Design review of the part built by this model. Coordinates are the model's own, in mm. A direction names the side the tool comes from. Round coordinates to 2 decimals unless told otherwise and drop trailing zeros. Order: outer loops, then holes, each group sorted by start corner. A loop starts at its lowest first (then second) coordinate and runs counter-clockwise, first axis right, second up.
from build123d import *

# Parameters (mm, degrees)
CROQUIS1_W              = 57
CROQUIS1_H              = 57
SALIENTE_EXTRUIR1_DEPTH = 18
REDONDEO1_R             = 5
CROQUIS2_W              = 14
CROQUIS2_H              = 10
CORTAR_EXTRUIR1_DEPTH   = 5


with BuildPart() as part:
    # Croquis1 → Saliente-Extruir1 (new body)
    with BuildSketch(Plane(origin=(0, 0, 0), x_dir=(1, 0, 0), z_dir=(0, 1, 0))):
        Rectangle(CROQUIS1_W, CROQUIS1_H)
    extrude(amount=SALIENTE_EXTRUIR1_DEPTH)

    # Redondeo1
    redondeo1_edges = [part.edges().sort_by_distance(p)[0] for p in [
        (-28.5, 9, -28.5),
        (28.5, 9, -28.5),
        (28.5, 9, 28.5),
        (-28.5, 9, 28.5),
    ]]
    fillet(redondeo1_edges, radius=REDONDEO1_R)

    # Croquis2 → Cortar-Extruir1 (cut)
    with BuildSketch(Plane(origin=(28.5, 0, 0), x_dir=(0, 0, -1), z_dir=(1, 0, 0))):
        with BuildLine():
            Line((-13, 12.5), (-7, 12.5))
            ThreePointArc((-7, 12.5), (-3.5, 9), (-7, 5.5))
            Line((-7, 5.5), (-13, 5.5))
            ThreePointArc((-13, 5.5), (-16.5, 9), (-13, 12.5))
        make_face()
        with Locations((10.5, 9)):
            Rectangle(CROQUIS2_W, CROQUIS2_H)
    extrude(amount=-CORTAR_EXTRUIR1_DEPTH, mode=Mode.SUBTRACT)


solid = part.part
1) Clearance check with flat-ended pins moving along their axes: P1, Ø1.5, axis at x = 26, y = 11, coming from the +Z side; P2, Ø3.5, axis at y = 10.5, z = 11, coming from the +X side; P3, Ø4, axis at x = 26.5, z = -12.5, coming from the -Y side; P4, Ø2.5, axis at x = 25.5, y = 11, coming from the -Z side. State where each tip first meets the part, or that it passes through.
Results:
P1: stops at z = 28.18
P2: stops at x = 23.5
P3: stops at y = 0
P4: stops at z = -28.44
2) For faces 1 (the face through (26, 8.9, 16.5)), 2 (the face through (0, 9, 28.5)), list the 3-axis set-ups (+Z, -Z, +X, -X, +Y, -Y) from which the entire face can be reached by the end or side of a thin tool; tool diameter is ignored.
Results:
face 1: +X
face 2: +Z, +X, -X, +Y, -Y
3) To check wall thickness, follow line 1 along X through (y, z) = (12, 11.5); line 2 along Z through (x, y) = (-25, 13.75); line 3 along Z through (x, y) = (24, 4.25). State the ranges of each line that lie inside material, in increasing order.
Results:
line 1: x = -28.5 to 23.5
line 2: z = -28.27 to 28.27
line 3: z = -28.47 to -17.5, -3.5 to 28.47
4) Take a section at A-A on z = 5. Give the boundary of the cut face in (x, y).
Results:
outline: (-28.5, 0) - (28.5, 0) - (28.5, 6.13) - (23.5, 6.13) - (23.5, 11.87) - (28.5, 11.87) - (28.5, 18) - (-28.5, 18) - close
5) The part is to be moulded in two halves that separate along Y. For faces 3 (the face through (27.07, 9.13, -27)), 4 (the face through (23.5, 9, 10)), 5 (the face through (0, 18, 0)), 6 (the face through (26, 9.1, 3.5)), say which applies: released by +Y, released by -Y, zero draft, split by the parting line, or undercut.
Results:
face 3: zero draft
face 4: undercut
face 5: released by +Y
face 6: undercut
6) Take a section at B-B on x = 24.5. Give the boundary of the cut face in (y, z), plus the area to 3 significant figures.
Results:
outline: (0, -28.4) - (18, -28.4) - (18, 28.4) - (0, 28.4) - close; hole (4, -17.5) - (14, -17.5) - (14, -3.5) - (4, -3.5) - close; hole (5.5, 7) arc R3.5 ccw to (12.5, 7) - (12.5, 13) arc R3.5 ccw to (5.5, 13) - close
area: 802 mm2
7) Take a section at C-C on y = 9. Give the boundary of the cut face in (x, z), plus the area to 3 significant figures.
Results:
outline: (-28.5, -23.5) arc R5 ccw to (-23.5, -28.5) - (23.5, -28.5) arc R5 ccw to (28.5, -23.5) - (28.5, -17.5) - (23.5, -17.5) - (23.5, -3.5) - (28.5, -3.5) - (28.5, 3.5) - (23.5, 3.5) - (23.5, 16.5) - (28.5, 16.5) - (28.5, 23.5) arc R5 ccw to (23.5, 28.5) - (-23.5, 28.5) arc R5 ccw to (-28.5, 23.5) - close
area: 3,090 mm2
